Print and shaded views of the part. All mm, measured from the part's lowest x, y and z. A direction names the side the tool comes from. Round coordinates to 2 decimals unless told otherwise and drop trailing zeros. Loops run counter-clockwise (first coordinate to the right, second up) from the corner with the lowest first, then second, coordinate; pieces in that order, holes last. Notation, with made-up numbers: (18, -32) -> (28, -32) arc R15 ccw to (28, -4) -> close; hole circle Ø3 at (38, 46.25). An arc over 180 degrees is marked (long way). Answer as CSV lines item,"result".
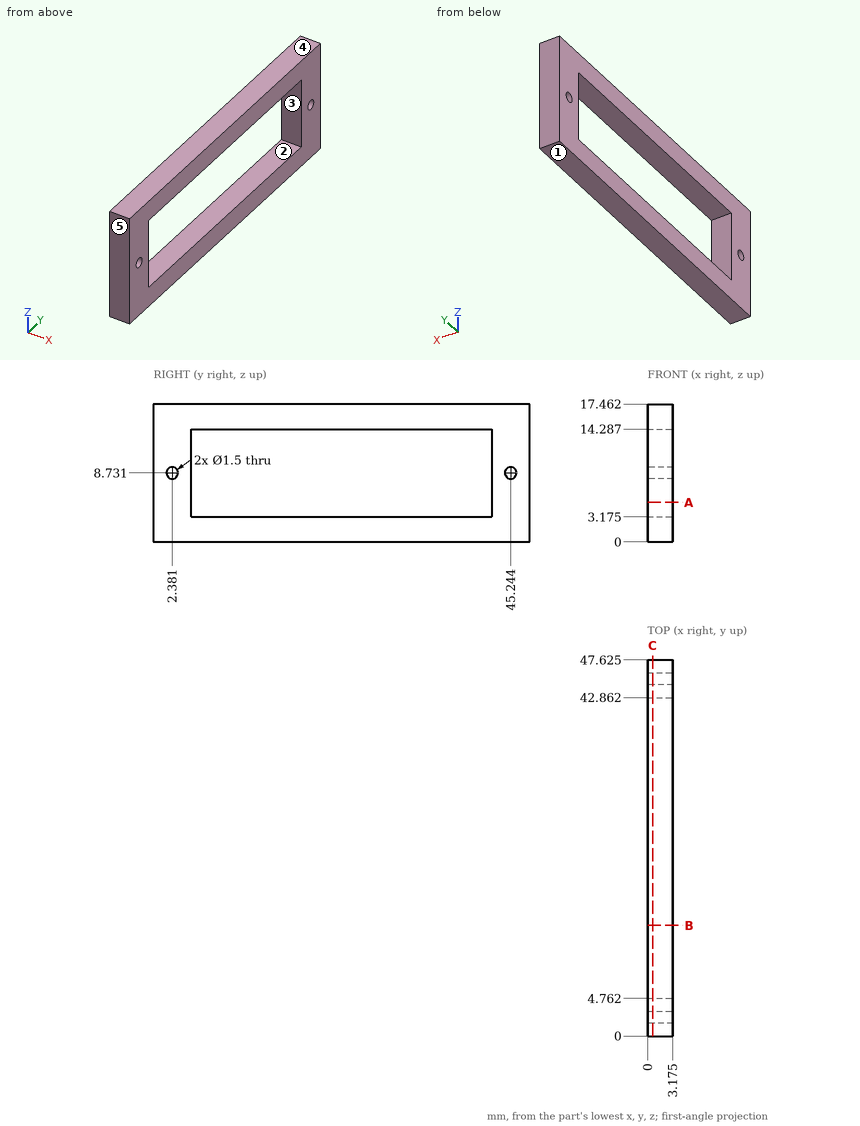
Q1. Drop flat-ended pins along their axis: pin 1 Ø2 at (y, z) = (40.5, 10.5) entering from -X; pin 2 Ø1.6 at (x, z) = (1, 11.5) entering from -Y. Give the stop position or say it passes through.
Results:
pin 1,"through"
pin 2,"y = 0"
Q2. Probe L1, parallel to Y at x = 1.7, z = 8.75 (1 decimal); L2, parallel to Z at x = 1.8, y = 5 (1 decimal); L3, parallel to Y at x = 2.65, z = 13 (1 decimal). List the from-to ranges inside material, lowest first. Write a range as [from, to].
Results:
L1,"[0, 1.6], [3.1, 4.8], [42.9, 44.5], [46, 47.6]"
L2,"[0, 3.2], [14.3, 17.5]"
L3,"[0, 4.8], [42.9, 47.6]"
Q3. Two-plate mould, pull along Z, no slides. Class the marked faces 3, 4 and 5: pulls with the +Z half, pulls with the -Z half, needs draft (parallel to the pull), parting line crosses it, or undercut.
Results:
face 3,"undercut"
face 4,"pulls with the +Z half"
face 5,"needs draft"
Q4. Slice it at C-C, the plane x = 0.65. Count the separate pieces of the cut face and the enclosed holes in it.
Results:
separate pieces,"1"
enclosed holes,"3"
Q5. Slice it at B-B, the plane y = 14. Give the cut face in (x, z) (1 decimal).
Results:
outline,"(0, 0) -> (3.2, 0) -> (3.2, 3.2) -> (0, 3.2) -> close; (0, 14.3) -> (3.2, 14.3) -> (3.2, 17.5) -> (0, 17.5) -> close"
Q6. Slice it at A-A, the plane z = 5. Give the cut face in (x, y) (1 decimal).
Results:
outline,"(0, 0) -> (3.2, 0) -> (3.2, 4.8) -> (0, 4.8) -> close; (0, 42.9) -> (3.2, 42.9) -> (3.2, 47.6) -> (0, 47.6) -> close"
Q7. Tool access for the marked faces 1 and 2: list every direction of +Z, -Z, +X, -X, +Y, -Y with a clear straight run to the whole face (end or side of a thin tool).
Results:
face 1,"-Z, +X, -X, +Y, -Y"
face 2,"+X, -X"
